Part model, mm, in its own coordinate system. Face numbers are marked on the shaded views. A direction names the side the tool comes from. Give positions to 0.01 mm unless a question says otherwise; leave off trailing zeros. Order: outer loops, then holes, each group sorted by start corner. A loop starts at its lowest first (then second) coordinate and runs counter-clockwise, first axis right, second up. Notation, with made-up numbers: M 21,32 L 67,32 A17 ccw 67,64 Z; hole C 70,23 d9. An arc over 180 degrees is marked long. One line per question, with ' | ' between items.
```python
from build123d import *

# Parameters (mm, degrees)
CUT_REVOLVE_1_ANGLE      = 50
PATTERN_CIRCULAR_1_COUNT = 3


with BuildPart() as part:
    # 草图1 → 旋转1 (revolve)
    with BuildSketch(Plane.XY):
        with BuildLine():
            Line((0, 37.5), (0, 46.5))
            Line((0, 46.5), (6.25, 46.5))
            Line((6.25, 46.5), (6.25, 42.037929302))
            ThreePointArc((6.25, 42.037929302), (30.49459553, 29.60286546), (42.20485754, 5))
            Line((42.20485754, 5), (50, 5))
            Line((50, 5), (50, 0))
            Line((50, 0), (37.5, 0))
            ThreePointArc((37.5, 0), (26.516504294, 26.516504294), (0, 37.5))
        make_face()
    revolve(axis=Axis((0, 37.5, 0), (0, 1, 0)))

    # 草图2 → 切除-旋转1 (revolve, symmetric, cut)
    with BuildSketch(Plane.XY) as cut_revolve_1_sk:
        with BuildLine():
            Line((15, 39.764934301), (15, 34.369317712))
            ThreePointArc((15, 34.369317712), (28.325677697, 24.574498632), (36.142080737, 10))
            Line((36.142080737, 10), (41.306779105, 10))
            ThreePointArc((41.306779105, 10), (31.844955201, 28.145138625), (15, 39.764934301))
        make_face()
    cut_revolve_1 = revolve(axis=Axis((0, 61.674672097, 0), (0, -1, 0)), revolution_arc=CUT_REVOLVE_1_ANGLE / 2, mode=Mode.SUBTRACT)
    cut_revolve_1 = cut_revolve_1 + revolve(cut_revolve_1_sk.sketch, axis=Axis((0, 61.674672097, 0), (0, 1, 0)), revolution_arc=CUT_REVOLVE_1_ANGLE / 2, mode=Mode.SUBTRACT)

    # 阵列(圆周)1: 切除-旋转1 ×3 about axis
    pattern_circular_1_axis = Axis((0, 0, 0), (0, 1, 0))
    for i in range(1, PATTERN_CIRCULAR_1_COUNT):
        add(cut_revolve_1.rotate(pattern_circular_1_axis, i * 360 / PATTERN_CIRCULAR_1_COUNT), mode=Mode.SUBTRACT)


solid = part.part
```
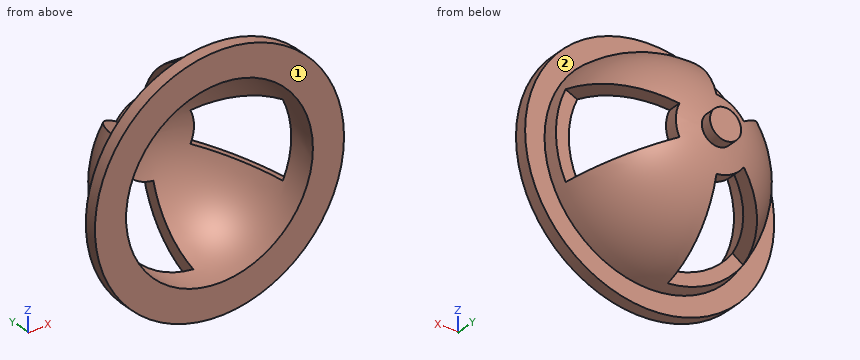
1. Slice it at B-B on z = 4.5. Give the cut face in (x, y).
Worked out:
outline: M -49.8,0 L -37.23,0 A37.23 cw 14.31,34.37 L 14.31,39.76 A42.26 ccw 4.34,42.04 L 4.34,46.5 L -4.34,46.5 L -4.34,42.04 A42.26 ccw -41.96,5 L -49.8,5 Z; M 35.86,10 A37.23 cw 37.23,0 L 49.8,0 L 49.8,5 L 41.96,5 A42.26 ccw 41.06,10 Z
2. Slice it at C-C on x = 18. Give the cut face in (y, z).
Worked out:
outline: M 0,-46.65 L 5,-46.65 L 5,-38.17 A38.5 ccw 37.57,-8.39 L 31.81,-8.39 A32.9 cw 0,-32.9 Z; M 0,32.9 A32.9 cw 31.81,8.39 L 37.57,8.39 A38.5 ccw 5,38.17 L 5,46.65 L 0,46.65 Z
3. Probe L1, parallel to Y at x = -24, z = 33.5; L2, parallel to Y at x = -18.5, z = 42; L3, parallel to Z at x = 8, y = 22.5. List the from-to ranges inside material, lowest first. Write a range as from..to.
Worked out:
L1: y = 0..10 | L2: y = 0..5 | L3: z = -35.16..-28.91, 28.91..35.16
4. Slice it at A-A on y = 11.5. Give the cut face in (x, z).
Worked out:
outline: M -33.52,-23.47 L -29.24,-20.47 A35.69 cw -29.24,20.47 L -33.52,23.47 A40.91 ccw Z; M -3.57,-40.76 A40.91 ccw 37.08,-17.29 L 32.35,-15.08 A35.69 cw -3.11,-35.56 Z; M -3.57,40.76 L -3.11,35.56 A35.69 cw 32.35,15.08 L 37.08,17.29 A40.91 ccw Z
5. Tool access for the marked faces 1 and 2: list every direction of +Z, -Z, +X, -X, +Y, -Y with a clear straight run to the whole face (end or side of a thin tool).
Worked out:
face 1: +Z, -Z, +X, -X, -Y | face 2: +Y
6. Slice it at D-D on x = 0. Give the cut face in (y, z).
Worked out:
outline: M 0,-50 L 5,-50 L 5,-42.2 A42.5 ccw 42.04,-6.25 L 46.5,-6.25 L 46.5,6.25 L 42.04,6.25 A42.5 ccw 5,42.2 L 5,50 L 0,50 L 0,37.5 A37.5 cw 0,-37.5 Z
7. Drop flat-ended pins along their axis: pin 1 (22.5 mm diameter, centred on x = -24.5, z = 28, fed in from +Y); pin 2 (22.5 mm diameter, centred on x = -22.5, z = -32, fed in from +Y); pin 3 (12 mm diameter, centred on y = 13, z = -38, fed in from +X). Give the stop position or say it passes through.
Worked out:
pin 1: stops at y = 30.86 | pin 2: stops at y = 10 | pin 3: stops at x = 25.28
